from build123d import *

# Parameters (mm, degrees)
BOSS_EXTRUDE1_DEPTH   = 6.35
M6_TAPPED_HOLE1_D     = 5
M6_TAPPED_HOLE1_DEPTH = 25.4
M6_TAPPED_HOLE1_TIP   = 1.502151548
M6_TAPPED_HOLE2_D     = 5
CUT_EXTRUDE1_DEPTH    = 88.888124909


with BuildPart() as part:
    # Sketch1 → Boss-Extrude1 (new, symmetric)
    with BuildSketch(Plane(origin=(0, 0, 0), x_dir=(0, 0, -1), z_dir=(1, 0, 0))):
        with BuildLine():
            Line((0, 0), (78, 0))
            Line((78, 0), (78, 58))
            Line((78, 58), (62, 58))
            Line((62, 58), (62, 28))
            ThreePointArc((62, 28), (59.071067812, 20.928932188), (52, 18))
            Line((52, 18), (0, 18))
            Line((0, 18), (0, 0))
        make_face()
    extrude(amount=BOSS_EXTRUDE1_DEPTH, both=True)

    # M6 Tapped Hole1
    with Locations(Plane(origin=(0, 0, -78), x_dir=(-1, 0, 0), z_dir=(0, 0, -1))):
        with Locations((0, 9), (0, 36)):
            Hole(M6_TAPPED_HOLE1_D / 2, depth=M6_TAPPED_HOLE1_DEPTH)
            with Locations((0, 0, -(M6_TAPPED_HOLE1_DEPTH + M6_TAPPED_HOLE1_TIP / 2))):  # 118° drill point
                Cone(0, M6_TAPPED_HOLE1_D / 2, M6_TAPPED_HOLE1_TIP, mode=Mode.SUBTRACT)

    # M6 Tapped Hole2 (through all)
    with Locations(Plane(origin=(0, 0, -78), x_dir=(-1, 0, 0), z_dir=(0, 0, -1))):
        with Locations((0, 52)):
            Hole(M6_TAPPED_HOLE2_D / 2)

    # Sketch4 → Cut-Extrude1 (cut, through all)
    with BuildSketch(Plane(origin=(0, 18, 0), x_dir=(1, 0, 0), z_dir=(0, 1, 0))):
        with BuildLine():
            Line((3.3, 45.45), (3.3, 38.55))
            ThreePointArc((3.3, 38.55), (0, 35.25), (-3.3, 38.55))
            Line((-3.3, 38.55), (-3.3, 45.45))
            ThreePointArc((-3.3, 45.45), (0, 48.75), (3.3, 45.45))
        make_face()
        with BuildLine():
            Line((3.3, 21.45), (3.3, 14.55))
            ThreePointArc((3.3, 14.55), (0, 11.25), (-3.3, 14.55))
            Line((-3.3, 14.55), (-3.3, 21.45))
            ThreePointArc((-3.3, 21.45), (0, 24.75), (3.3, 21.45))
        make_face()
    extrude(amount=-CUT_EXTRUDE1_DEPTH, mode=Mode.SUBTRACT)


solid = part.part
Source: CAD feature listing. Evaluate the final solid. Frame: model axes, mm. A direction names the side the tool comes from. Round coordinates to 2 decimals unless told otherwise and drop trailing zeros. Loops run counter-clockwise (first coordinate to the right, second up) from the corner with the lowest first, then second, coordinate; pieces in that order, holes last. Notation, with made-up numbers: (-15.75, 6.25) - (37.25, 6.25) arc R14 cw to (37.25, 33.25) - close; hole circle Ø4 at (76, -31.5). An arc over 180 degrees is marked (long way). Write item = value, one per line. Start each with the question number.
Item 1: Mould query, pull axis Y, two halves, no side actions, for faces 4 (the face through (-0.23, 9.37, -51.36)), 5 (the face through (0, 18, -26)), 6 (the face through (-0.07, 9.13, -24.75)), 7 (the face through (-0.54, 6.56, -65.12)). Classes: released by +Y, released by -Y, zero draft, split by the parting line, or undercut.
Item 2: Section query D-D on y = 29. Output: boundary loops of the cut face in (x, z), plus the area to 3 significant figures.
Item 3: First-contact query: pin 1 Ø4 at (x, z) = (-2, -35) entering from +Y; pin 2 Ø2 at (x, y) = (-1, 39) entering from +Z. Flat tips, straight axial feed; report the tip coordinate or a pass-through.
Item 4: Reachability of faces 1 (the face through (0, 43, -62)), 2 (the face through (4, 0, -38)), 3 (the face through (0.07, 9.13, -11.25)) from +Z, -Z, +X, -X, +Y, -Y: full face, straight path, thin tool, end or side. Return the list, or none.
Item 5: Section query B-B on z = -72. Output: boundary loops of the cut face in (x, y), plus the area to 3 significant figures.
Item 6: Section query C-C on x = -4.5. Output: boundary loops of the cut face in (y, z), plus the area to 3 significant figures.
Item 7: Material intervals for line 1 (Y direction, x = 0, z = -72.5); line 2 (Y direction, x = -2.25, z = -65); line 3 (X direction, y = 9, z = -65.5), sorted ascending.
Item 8: Section query A-A on y = 52. Output: boundary loops of the cut face in (x, z), plus the area to 3 significant figures.
Results list:
q1.face_4 = undercut
q1.face_5 = released by +Y
q1.face_6 = zero draft
q1.face_7 = undercut
q2.outline = (-6.35, -78) - (6.35, -78) - (6.35, -62) - (-6.35, -62) - close
q2.area = 203 mm²
q3.pin_1 = 18
q3.pin_2 = -62
q4.face_1 = +Z, +X, -X, +Y
q4.face_2 = +Z, -Z, +X, -X, -Y
q4.face_3 = +Y, -Y
q5.outline = (-6.35, 0) - (6.35, 0) - (6.35, 58) - (-6.35, 58) - close; hole circle Ø5 at (0, 9); hole circle Ø5 at (0, 36); hole circle Ø5 at (0, 52)
q5.area = 678 mm²
q6.outline = (0, -78) - (58, -78) - (58, -62) - (28, -62) arc R10 cw to (18, -52) - (18, 0) - (0, 0) - close
q6.area = 2,070 mm²
q7.line_1 = 0 to 6.5, 11.5 to 33.5, 38.5 to 49.5, 54.5 to 58
q7.line_2 = 0 to 7.91, 10.09 to 34.91, 37.09 to 50.91, 53.09 to 58
q7.line_3 = -6.35 to -2.5, 2.5 to 6.35
q8.outline = (-6.35, -78) - (-2.5, -78) - (-2.5, -62) - (-6.35, -62) - close; (2.5, -78) - (6.35, -78) - (6.35, -62) - (2.5, -62) - close
q8.area = 123 mm²
